from build123d import *

# Parameters (mm, degrees)
SKETCH1_W                = 188.976
SKETCH1_H                = 34.29
BOSS_EXTRUDE1_DEPTH      = 12.954
CUT_EXTRUDE1_DEPTH       = 121.412
CUT_EXTRUDE2_DEPTH       = 25.4
SKETCH3_W                = 165.1
SKETCH3_H                = 11.176
CUT_EXTRUDE3_DEPTH       = 193.498152698
CUT_EXTRUDE4_DEPTH       = 25.4
SKETCH5_W                = 6.35
SKETCH5_H                = 90.424
CUT_EXTRUDE6_DEPTH       = 193.498152698
SKETCH5_4_W              = 6.35
SKETCH5_4_H              = 11.176
CUT_EXTRUDE7_DEPTH       = 10.414
CUT_EXTRUDE8_DEPTH       = 193.498152698
CUT_EXTRUDE9_DEPTH       = 193.17529886
CUT_EXTRUDE10_DEPTH      = 193.498152715
CUT_EXTRUDE10_DEPTH_BACK = 193.498152715
SKETCH12_W               = 2.54
SKETCH12_H               = 4.572
CUT_EXTRUDE12_DEPTH      = 67.31


with BuildPart() as part:
    # Sketch1 → Boss-Extrude1 (new body)
    with BuildSketch(Plane(origin=(0, 0, 0), x_dir=(0, 0, -1), z_dir=(1, 0, 0))):
        with Locations((94.488, 17.145)):
            Rectangle(SKETCH1_W, SKETCH1_H)
    extrude(amount=BOSS_EXTRUDE1_DEPTH)

    # Sketch2 → Cut-Extrude1 (cut)
    with BuildSketch(Plane.XY):
        with BuildLine():
            ThreePointArc((0, 31.496), (-6.35, 25.146), (0, 18.796))
            Line((0, 18.796), (0, 31.496))
        make_face()
        with BuildLine():
            Line((0, 31.496), (0, 18.796))
            ThreePointArc((0, 18.796), (4.490128061, 20.655871939), (6.35, 25.146))
            ThreePointArc((6.35, 25.146), (4.490128061, 29.636128061), (0, 31.496))
        make_face()
    extrude(amount=-CUT_EXTRUDE1_DEPTH, mode=Mode.SUBTRACT)

    # Sketch2_3 → Cut-Extrude2 (cut)
    with BuildSketch(Plane.XY):
        with BuildLine():
            ThreePointArc((0, 4.572), (1.975656347, 5.390343653), (2.794, 7.366))
            ThreePointArc((2.794, 7.366), (1.975656347, 9.341656347), (0, 10.16))
            Line((0, 10.16), (0, 4.572))
        make_face()
        with BuildLine():
            Line((0, 4.572), (0, 10.16))
            ThreePointArc((0, 10.16), (-2.794, 7.366), (0, 4.572))
        make_face()
    extrude(amount=-CUT_EXTRUDE2_DEPTH, mode=Mode.SUBTRACT)

    # Sketch3 → Cut-Extrude3 (cut, through all)
    with BuildSketch(Plane.ZY):
        with Locations((-106.426, 5.588)):
            Rectangle(SKETCH3_W, SKETCH3_H)
    extrude(amount=-CUT_EXTRUDE3_DEPTH, mode=Mode.SUBTRACT)

    # Sketch4 → Cut-Extrude4 (cut)
    with BuildSketch(Plane.XY):
        with BuildLine():
            Line((7.366, 11.176), (7.366, 7.366))
            ThreePointArc((7.366, 7.366), (5.20854855, 2.15745145), (0, 0))
            Line((0, 0), (12.954, 0))
            Line((12.954, 0), (12.954, 11.176))
            Line((12.954, 11.176), (7.366, 11.176))
        make_face()
    extrude(amount=-CUT_EXTRUDE4_DEPTH, mode=Mode.SUBTRACT)

    # Sketch5 → Cut-Extrude6 (cut, through all)
    with BuildSketch(Plane(origin=(0, 34.29, 0), x_dir=(1, 0, 0), z_dir=(0, 1, 0))):
        with Locations((3.175, 69.088)):
            Rectangle(SKETCH5_W, SKETCH5_H)
    extrude(amount=-CUT_EXTRUDE6_DEPTH, mode=Mode.SUBTRACT)

    # Sketch5_4 → Cut-Extrude7 (cut)
    with BuildSketch(Plane(origin=(0, 34.29, 0), x_dir=(1, 0, 0), z_dir=(0, 1, 0))):
        with Locations((3.175, 18.288)):
            Rectangle(SKETCH5_4_W, SKETCH5_4_H)
    extrude(amount=-CUT_EXTRUDE7_DEPTH, mode=Mode.SUBTRACT)

    # Sketch6 → Cut-Extrude8 (cut, through all)
    with BuildSketch(Plane.XY):
        with BuildLine():
            ThreePointArc((0, 34.29), (4.74341842, 32.963462356), (8.110563197, 29.368736153))
            Line((8.110563197, 29.368736153), (12.954, 20.066))
            Line((12.954, 20.066), (12.954, 34.29))
            Line((12.954, 34.29), (0, 34.29))
        make_face()
    extrude(amount=-CUT_EXTRUDE8_DEPTH, mode=Mode.SUBTRACT)

    # Sketch7 → Cut-Extrude9 (cut, through all)
    with BuildSketch(Plane.ZY.offset(-6.35)):
        with BuildLine():
            Line((-33.207309556, 31.725531594), (-114.3, 31.725531594))
            Line((-114.3, 31.725531594), (-114.3, 25.146))
            Line((-114.3, 25.146), (-114.3, 23.876))
            Line((-114.3, 23.876), (-23.876, 23.876))
            Line((-23.876, 23.876), (-23.114000049, 23.876))
            ThreePointArc((-23.114000049, 23.876), (-29.507161288, 26.069362267), (-33.207309556, 31.725531594))
        make_face()
        with BuildLine():
            Line((-33.528, 34.29), (-114.3, 34.29))
            Line((-114.3, 34.29), (-114.3, 31.725531594))
            Line((-114.3, 31.725531594), (-33.207309556, 31.725531594))
            ThreePointArc((-33.207309556, 31.725531594), (-33.447516384, 32.997778989), (-33.528, 34.29))
        make_face()
        with BuildLine():
            Line((-13.020690444, 31.725531594), (-33.207309556, 31.725531594))
            ThreePointArc((-33.207309556, 31.725531594), (-29.507161288, 26.069362267), (-23.114000049, 23.876))
            ThreePointArc((-23.114000049, 23.876), (-16.72083875, 26.069362237), (-13.020690444, 31.725531594))
        make_face()
        with BuildLine():
            Line((-12.7, 34.29), (-33.528, 34.29))
            ThreePointArc((-33.528, 34.29), (-33.447516384, 32.997778989), (-33.207309556, 31.725531594))
            Line((-33.207309556, 31.725531594), (-13.020690444, 31.725531594))
            ThreePointArc((-13.020690444, 31.725531594), (-12.780483616, 32.997778989), (-12.7, 34.29))
        make_face()
    extrude(amount=-CUT_EXTRUDE9_DEPTH, mode=Mode.SUBTRACT)

    # Sketch8 → Cut-Extrude10 (cut, two sides: drawn at the far end of the back side and taken through both)
    with BuildSketch(Plane.ZY.offset(-CUT_EXTRUDE10_DEPTH_BACK)):
        Polygon((-188.976, 34.29), (-188.976, 11.176), (-180.103366694, 34.29), align=None)
    extrude(amount=CUT_EXTRUDE10_DEPTH + CUT_EXTRUDE10_DEPTH_BACK, mode=Mode.SUBTRACT)

    # Sketch12 → Cut-Extrude12 (cut)
    with BuildSketch(Plane.XY.offset(-188.976)):
        Polygon((8.382, 18.542), (0, 18.542), (0, 11.176), (8.382, 11.176), (8.382, 13.97), align=None)
        with Locations((9.652, 16.256)):
            Rectangle(SKETCH12_W, SKETCH12_H)
    extrude(amount=CUT_EXTRUDE12_DEPTH, mode=Mode.SUBTRACT)


solid = part.part
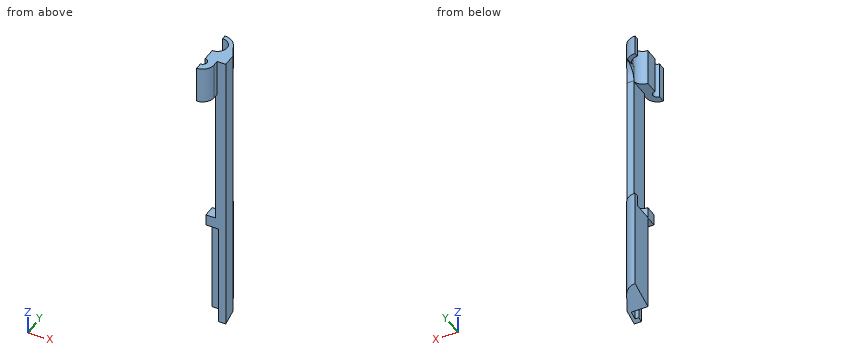
The listing builds one solid part. Answer for the finished solid, in the listing's coordinates (mm). Round coordinates to 2 decimals unless told otherwise and drop trailing zeros. Write each loop counter-clockwise with the first axis right and the second up, starting at its lowest first coordinate (ties: lowest second). Pieces come first, ordered by that corner, then holes. Notation, with made-up numbers: M 30,-16.75 L 63,-16.75 A12 ccw 63,4.25 Z; hole C 22,45 d1. An arc over 180 degrees is marked long. Write each question's results on one line, items separated by ' | '. Start each with the question number.
(1) The part is cut by section B-B, the plane y = 17. Write down the section's boundary in (x, z).
(2) Find the intervals of material crossed by line 1 (Z direction, x = 2.75, y = 15.5); line 2 (Y direction, x = 3.25, z = -8); line 3 (X direction, y = 16, z = -54), in increasing order.
(3) The part is cut by section A-A, the plane z = -171. Write down the section's boundary in (x, y), and give its area (3 significant figures).
(4) Each of these flat-tipped pins is pushed along its axis until it touches: P1, Ø3, axis at x = 4.5, y = 31.5, coming from the -Z side; P2, Ø1.5, axis at x = 5.5, y = 12, coming from the +Z side; P3, Ø6.5, axis at x = 4.5, z = -87, coming from the -Y side; P4, Ø1.3, axis at x = 10, z = -166.5, coming from the +Y side. Where does it stop, or does it pass through?
(5) The part is cut by section C-C, the plane z = -66. Write down the section's boundary in (x, y).
Worked answers:
1) outline: M 0,-121.67 L 10.92,-121.67 L 10.92,-186.74 L 12.95,-186.74 L 12.95,0 L 0,0 L 0,-23.88 L 6.35,-23.88 L 6.35,-114.3 L 0,-114.3 Z
2) line 1: z = -121.67 to -114.3, -23.88 to 0 | line 2: y = 0.76 to 19.69, 30.6 to 33.69 | line 3: x = 6.35 to 12.95
3) outline: M 0,18.54 L 10.92,18.54 L 10.92,13.97 L 8.38,13.97 L 8.38,11.18 L 12.95,11.18 L 12.95,20.07 L 8.11,29.37 A9.14 ccw 0,34.29 Z | area: 168 mm²
4) P1: stops at z = -181.75 | P2: stops at z = 0 | P3: stops at y = 11.18 | P4: stops at y = 26.99
5) outline: M 6.35,11.18 L 12.95,11.18 L 12.95,20.07 L 10.97,23.88 L 6.35,23.88 Z
